Design review of the part built by this model. Coordinates are the model's own, in mm. Face numbers are marked on the shaded views. A direction names the side the tool comes from. Give positions to 0.01 mm unless a question says otherwise; leave off trailing zeros. Write each loop counter-clockwise with the first axis right and the second up, starting at its lowest first coordinate (ties: lowest second). Pieces come first, ordered by that corner, then holes.
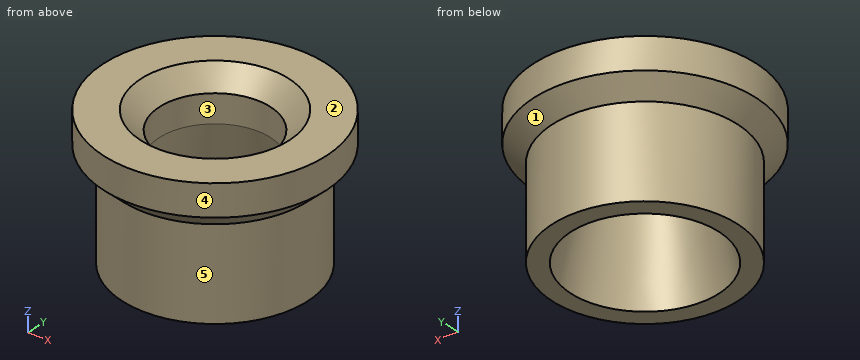
```python
from build123d import *

# Parameters (mm, degrees)
CROQUIS2_R            = 3
CORTAR_EXTRUIR1_DEPTH = 10
CHAFL_N1_SIZE         = 1


with BuildPart() as part:
    # Croquis1 → Revolución1 (revolve)
    with BuildSketch(Plane(origin=(0, 0, 0), x_dir=(1, 0, 0), z_dir=(0, 1, 0))):
        Polygon((-3, -1.25), (-4, 3.75), (-5, 3.75), (-5, -1.140510949), (-6, -2.062248439), (-6, -3.75), (0, -3.75), (0, -1.25), align=None)
    revolve(axis=Axis((0, 0, -3.75), (0, 0, 1)))

    # Croquis2 → Cortar-Extruir1 (cut)
    with BuildSketch(Plane.XY.offset(3.75)):
        Circle(CROQUIS2_R)
    extrude(amount=-CORTAR_EXTRUIR1_DEPTH, mode=Mode.SUBTRACT)

    # Chaflán1
    chafl_n1_edges = [part.edges().sort_by_distance(p)[0] for p in [
        (-3, 0, 3.75),
    ]]
    chamfer(chafl_n1_edges, length=CHAFL_N1_SIZE)


solid = part.part
```
(1) To check wall thickness, follow L1, parallel to Y at x = 0, z = 2.35; L2, parallel to X at y = -4, z = -0.5. State the ranges of each line that lie inside material, in increasing order.
Resolved:
L1: y = -6 to -3, 3 to 6
L2: x = -3 to 3
(2) Clearance check with flat-ended pins moving along their axes: P1, Ø5, axis at x = 0, y = 0, coming from the -Z side; P2, Ø1, axis at x = 1, z = 1, coming from the +Y side; P3, Ø3, axis at y = -4, z = 2, coming from the +X side; P4, Ø1, axis at x = 0.5, z = 0, coming from the -Y side. State where each tip first meets the part, or that it passes through.
Resolved:
P1: passes through
P2: stops at y = 5.3
P3: stops at x = 5.45
P4: stops at y = -5
(3) Consider section C-C, the plane z = 0. Give the boundary of the cut face in (x, y), then the cut area to 3 significant figures.
Resolved:
outline: circle Ø10 at (0, 0); hole circle Ø6.5 at (0, 0)
area: 45.4 mm2
(4) Consider section A-A, the plane y = 0. Give the boundary of the cut face in (x, z).
Resolved:
outline: (-6, 2.06) - (-5, 1.14) - (-5, -3.75) - (-4, -3.75) - (-3, 1.25) - (-3, 2.75) - (-4, 3.75) - (-6, 3.75) - close; (3, 1.25) - (4, -3.75) - (5, -3.75) - (5, 1.14) - (6, 2.06) - (6, 3.75) - (4, 3.75) - (3, 2.75) - close
(5) Consider section D-D, the plane z = -1.75. Give the boundary of the cut face in (x, y), then the cut area to 3 significant figures.
Resolved:
outline: circle Ø10 at (0, 0); hole circle Ø7.2 at (0, 0)
area: 37.8 mm2
(6) Tool access review of the marked faces 4 and 5: name each direction out of +Z, -Z, +X, -X, +Y, -Y from which nothing blocks a thin tool from reaching the whole face with its end or side.
Resolved:
face 4: +Z, -Z
face 5: -Z
(7) Mouldability with a two-part tool opening along X and no side actions: class the marked faces 1, 2 and 3 as pulls with the +X half, pulls with the -X half, needs draft (parallel to the pull), parting line crosses it, or undercut.
Resolved:
face 1: parting line crosses it
face 2: needs draft
face 3: undercut
